Read the model definition and answer for the solid it produces. Units are mm, in the model's axes. Face numbers are marked on the shaded views. A direction names the side the tool comes from. Coordinates: 2 decimals unless noted, no trailing zeros. Order: outer loops, then holes, each group sorted by start corner. A loop starts at its lowest first (then second) coordinate and runs counter-clockwise, first axis right, second up. Notation, with made-up numbers: (75, 53) -> (121, 53) arc R36 ccw to (121, 92) -> close; hole circle Ø4 at (46.5, 82.25). An arc over 180 degrees is marked (long way). Answer in a Markdown table with one row per item.
from build123d import *

# Parameters (mm, degrees)
SKETCH1_W           = 200
SKETCH1_H           = 200
BOSS_EXTRUDE1_DEPTH = 10
SKETCH2_R           = 20
BOSS_EXTRUDE2_DEPTH = 90


with BuildPart() as part:
    # Sketch1 → Boss-Extrude1 (new body)
    with BuildSketch(Plane.XY):
        with Locations((-2.425876011, -32.884097035)):
            Rectangle(SKETCH1_W, SKETCH1_H)
    extrude(amount=BOSS_EXTRUDE1_DEPTH)

    # Sketch2 → Boss-Extrude2 (add)
    with BuildSketch(Plane(origin=(0, 0, 0), x_dir=(-1, 0, 0), z_dir=(0, 0, -1))):
        with Locations((2.425876011, -32.884097035)):
            Circle(SKETCH2_R)
    extrude(amount=BOSS_EXTRUDE2_DEPTH)


solid = part.part
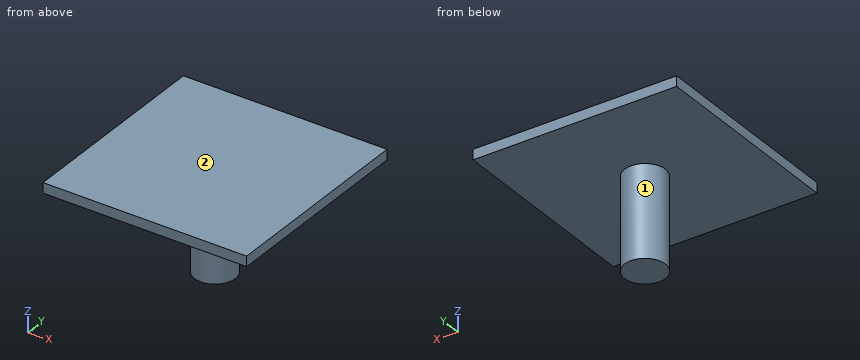
Q1. The part is cut by section C-C (z = -79). Write down the section's boundary in (x, y).
Outcome:
| item | result |
|---|---|
| outline | circle Ø40 at (-2.43, -32.88) |
Q2. The part is cut by section D-D (y = -63). Write down the section's boundary in (x, z).
Outcome:
| item | result |
|---|---|
| outline | (-102.43, 0) -> (97.57, 0) -> (97.57, 10) -> (-102.43, 10) -> close |
Q3. The part is cut by section B-B (y = -35.5). Write down the section's boundary in (x, z).
Outcome:
| item | result |
|---|---|
| outline | (-102.43, 0) -> (-22.25, 0) -> (-22.25, -90) -> (17.4, -90) -> (17.4, 0) -> (97.57, 0) -> (97.57, 10) -> (-102.43, 10) -> close |
Q4. Given pin 1 (3 mm diameter, centred on x = 8, z = -35.5, fed in from -Y); pin 2 (8 mm diameter, centred on y = -57.5, z = -52, fed in from +X), each flat-ended and moving along its own axis, determine where each tip first touches the part or whether it passes through.
Outcome:
| item | result |
|---|---|
| pin 1 | y = -50.78 |
| pin 2 | through |
Q5. Consider line 1 (Z direction, x = -66, y = 23.5); line 2 (Y direction, x = 13.5, z = -84); line 3 (Y direction, x = -9, z = -32.5). Determine where each line is inside the solid, lowest interval first.
Outcome:
| item | result |
|---|---|
| line 1 | 0 to 10 |
| line 2 | -44.98 to -20.79 |
| line 3 | -51.77 to -14 |
Q6. For the marked faces 1 and 2, determine the directions among +Z, -Z, +X, -X, +Y, -Y from which every point of the face is accessible in a straight line to the end or side of a thin tool.
Outcome:
| item | result |
|---|---|
| face 1 | -Z |
| face 2 | +Z, +X, -X, +Y, -Y |
Q7. The part is cut by section A-A (x = -54). Write down the section's boundary in (y, z), then the cut area to 3 significant figures.
Outcome:
| item | result |
|---|---|
| outline | (-132.88, 0) -> (67.12, 0) -> (67.12, 10) -> (-132.88, 10) -> close |
| area | 2,000 mm² |
